For this review, take the finished solid that the model builds, in its own axes (mm). Round coordinates to 2 decimals unless told otherwise and drop trailing zeros. Loops run counter-clockwise (first coordinate to the right, second up) from the corner with the lowest first, then second, coordinate; pieces in that order, holes last. Notation, with made-up numbers: (22, -26) -> (54, -26) arc R19 ccw to (54, -3) -> close; hole circle Ø1 at (65, 70.25). An arc over 180 degrees is marked (long way). Write each question's results on one line, items separated by ' | '.
```python
from build123d import *

# Parameters (mm, degrees)
SKETCH1_W               = 20
SKETCH1_H               = 6
BOSS_EXTRUDE1_DEPTH     = 4
CUT_EXTRUDE1_DEPTH      = 22.260291625
CUT_EXTRUDE1_DEPTH_BACK = 22.260291625
SKETCH2_R               = 1.45
FILLET1_R               = 3


with BuildPart() as part:
    # Sketch1 → Boss-Extrude1 (new body)
    with BuildSketch(Plane.XY):
        with Locations((10, -3)):
            Rectangle(SKETCH1_W, SKETCH1_H)
    extrude(amount=BOSS_EXTRUDE1_DEPTH)

    # Sketch2 → Cut-Extrude1 (cut, two sides: drawn at the far end of the back side and taken through both)
    with BuildSketch(Plane.XY.offset(4).offset(-CUT_EXTRUDE1_DEPTH_BACK)):
        with Locations((3, -3)):
            Circle(SKETCH2_R)
        with Locations((17, -3)):
            Circle(SKETCH2_R)
    extrude(amount=CUT_EXTRUDE1_DEPTH + CUT_EXTRUDE1_DEPTH_BACK, mode=Mode.SUBTRACT)

    # Fillet1
    fillet1_edges = [part.edges().sort_by_distance(p)[0] for p in [
        (20, -6, 2),
        (20, 0, 2),
        (0, -6, 2),
        (0, 0, 2),
    ]]
    fillet(fillet1_edges, radius=FILLET1_R - 0.0001)  # a hair under: the kernel refuses the full size


solid = part.part
```
1. Consider section B-B (y = -3.2). State the section outline as (x, z) points.
Values found:
outline: (0.01, 0) -> (1.56, 0) -> (1.56, 4) -> (0.01, 4) -> close; (4.44, 0) -> (15.56, 0) -> (15.56, 4) -> (4.44, 4) -> close; (18.44, 0) -> (19.99, 0) -> (19.99, 4) -> (18.44, 4) -> close
2. Consider section C-C (x = 17.75). State the section outline as (y, z) points, plus the area to 3 significant figures.
Values found:
outline: (-5.9, 0) -> (-4.24, 0) -> (-4.24, 4) -> (-5.9, 4) -> close; (-1.76, 0) -> (-0.1, 0) -> (-0.1, 4) -> (-1.76, 4) -> close | area: 13.3 mm2
3. Draft analysis for pull direction X (two halves, no side actions). For faces 1 (the face through (10, 0, 2)), 2 (the face through (1.55, -2.94, 1.97)), 3 (the face through (19.1, -0.86, 2.03)), state which applies: released by +X, released by -X, zero draft, split by the parting line, or undercut.
Values found:
face 1: zero draft | face 2: undercut | face 3: released by +X
4. Consider section A-A (z = 1.65). Give the number of separate pieces and of enclosed holes in the cut face, plus the area to 3 significant figures.
Values found:
separate pieces: 1 | enclosed holes: 2 | area: 99.1 mm2
5. Consider section D-D (y = -2.15). State the section outline as (x, z) points.
Values found:
outline: (0.12, 0) -> (1.83, 0) -> (1.83, 4) -> (0.12, 4) -> close; (4.17, 0) -> (15.83, 0) -> (15.83, 4) -> (4.17, 4) -> close; (18.17, 0) -> (19.88, 0) -> (19.88, 4) -> (18.17, 4) -> close
6. For pin 1 (1 mm diameter, centred on y = -4.5, z = 3.5, fed in from +X), flat-tipped, find the tip position at first contact; note if it passes through.
Values found:
pin 1: stops at x = 19.83
7. To check wall thickness, follow probe 1 along X at (y, z) = (-3, 2.45); probe 2 along Y at (x, z) = (3, 3.2); probe 3 along X at (y, z) = (-4.25, 2.5). State the ranges of each line that lie inside material, in increasing order.
Values found:
probe 1: x = 0 to 1.55, 4.45 to 15.55, 18.45 to 20 | probe 2: y = -6 to -4.45, -1.55 to 0 | probe 3: x = 0.27 to 2.27, 3.73 to 16.27, 17.73 to 19.73
